Source: CAD feature listing. Evaluate the final solid. Frame: model axes, mm. Give positions to 0.01 mm unless a question says otherwise; leave off trailing zeros. Order: outer loops, then holes, each group sorted by start corner. A loop starts at its lowest first (then second) coordinate and runs counter-clockwise, first axis right, second up. Notation, with made-up numbers: M 5.25,48.5 L 30.25,48.5 A30 cw 30.25,74.5 Z; hole C -20,86.5 d4. An arc over 180 degrees is marked long. Use CSV: the item, a comma, the result in double quotes. Start each with the question number.
Item 1: Section query B-B on y = -2.5. Return loops of the section in (x, z).
Item 2: Section query C-C on x = 18.35. Return loops of the section in (y, z).
Item 3: Ray query, probe 1 along Z at (x, y) = (18.55, -1.5); probe 2 along Z at (x, y) = (18.65, 3.5); probe 3 along Y at (x, z) = (18.65, 12.25). Return the intervals inside material, ascending. Write a range as from..to.
Item 4: Pull-direction query (Z, two-part tool) for faces 1 (the face through (18.5, -1.07, 6.31)), 2 (the face through (18.222, 1, 6)), 3 (the face through (18.504, 0.226, 15.764)); classes: +Z half, -Z half, draft (parallel to the pull), parting line (faces both ways), or undercut.
Item 5: Section query A-A on z = 14. Return loops of the section in (x, y).
Item 6: Section query D-D on z = 15.25. Return loops of the section in (x, y), and give its area (3 significant figures).
from build123d import *

# Parameters (mm, degrees)
SKETCH1_R           = 0.6
BOSS_EXTRUDE1_DEPTH = 1
SCALE1_SCALE        = 0.555555556


with BuildPart() as part:
    # Sketch1 → Boss-Extrude1 (new body)
    with BuildSketch(Plane(origin=(19, 0, 0), x_dir=(0, 0, -1), z_dir=(1, 0, 0))):
        with BuildLine():
            Line((-1.082906578, 1.214226965), (-0.806260325, 1.444819657))
            ThreePointArc((-0.806260325, 1.444819657), (-0.157167996, 2.46989624), (-0.220083072, 3.681566388))
            ThreePointArc((-0.220083072, 3.681566388), (-20.449170804, -0.000103807), (-0.220095755, -3.681843689))
            ThreePointArc((-0.220095755, -3.681843689), (-0.157177378, -2.470170425), (-0.806270581, -1.44509051))
            Line((-0.806270581, -1.44509051), (-1.082193901, -1.213563353))
            ThreePointArc((-1.082193901, -1.213563353), (-3.437745717, -1.969386585), (-1.886859109, -3.896727719))
            ThreePointArc((-1.886859109, -3.896727719), (-18.999593972, -0.000121806), (-1.886859109, 3.896484108))
            ThreePointArc((-1.886859109, 3.896484108), (-3.437385157, 1.97013231), (-1.082906578, 1.214226965))
        make_face()
        with Locations(Location((-2.00000003, -2.4, 0), (0, 0, 180))):
            Circle(SKETCH1_R, mode=Mode.SUBTRACT)
        with Locations(Location((-2.00000003, 2.4, 0), (0, 0, 180))):
            Circle(SKETCH1_R, mode=Mode.SUBTRACT)
    extrude(amount=-BOSS_EXTRUDE1_DEPTH)


with BuildPart() as part_1:
    # Scale1: scaled about (18.5, -0.000178585, 9.916688181)
    add(part.part.scale(SCALE1_SCALE).moved(Location((8.222222222, -7.9371e-05, 4.407416969))))


solid = part_1.part
Verdict:
1,outline,"M 18.22,4.72 L 18.78,4.72 L 18.78,5.63 L 18.22,5.63 Z; M 18.22,14.29 L 18.78,14.29 L 18.78,15.2 L 18.22,15.2 Z"
2,outline,"M -2.16,5.46 A5 cw long 2.16,5.46 A0.83 ccw long 0.67,5.01 L 0.8,4.86 A1.11 ccw 2.05,4.53 A5.81 ccw long -2.05,4.53 A1.11 ccw -0.8,4.86 L -0.67,5.01 A0.83 ccw long Z; hole C -1.33,5.52 d0.67; hole C 1.33,5.52 d0.67"
3,probe 1,"4.47..5.23, 5.81..6.34, 14.73..15.57"
3,probe 2,"5.33..6.39, 13.53..14.59"
3,probe 3,"-5.34..-4.45, 4.45..5.34"
4,face 1,"undercut"
4,face 2,"draft"
4,face 3,"parting line"
5,outline,"M 18.22,-4.17 L 18.78,-4.17 L 18.78,-2.95 L 18.22,-2.95 Z; M 18.22,2.95 L 18.78,2.95 L 18.78,4.17 L 18.22,4.17 Z"
6,outline,"M 18.22,-2.4 L 18.78,-2.4 L 18.78,2.4 L 18.22,2.4 Z"
6,area,"2.66 mm2"
